Autodesk Inventor part; units mm, degrees
ref_plane "YZ Plane" through (0, 0, 0) normal (1, 0, 0) x (0, 1, 0)
ref_plane "XZ Plane" through (0, 0, 0) normal (0, 1, 0) x (-1, 0, 0)
ref_plane "XY Plane" through (0, 0, 0) normal (0, 0, 1) x (1, 0, 0)
sketch "Skizze1" plane through (0, 0, 0) normal (0, 0, 1) x (1, 0, 0)
  line L0 (-68.016, 1.808) -> (67.584, 1.808)
  line L1 (67.584, 1.808) -> (67.584, -2.192)
  line L2 (67.584, -2.192) -> (-68.016, -2.192)
  line L3 (-68.016, -2.192) -> (-68.016, 1.808)
  line L4 (-68.016, 1.808) -> (67.584, -2.192) construction
  line L5 (67.584, 1.808) -> (-68.016, -2.192) construction
  point P0 (0, 0)
  point P1 (-0.216, -0.192)
  point P2 (-0.216, -0.192)
  dimension "d0" = 135.6
  dimension "d1" = 4
extrude "Extrusion1" add sketch "Skizze1" along normal mid plane 3.25
ref_plane "Arbeitsebene1" through (-68.016, -0.192, 1.625) normal (0, -1, 0) x (1, 0, 0)
sketch "Skizze2" plane through (-68.016, -0.192, 1.625) normal (0, -1, 0) x (1, 0, 0)
  line L0 (0, -3.25) -> (0, 0)
  line L1 (0, -3.25) -> (135.6, -3.25)
  line L2 (0, 0) -> (2.85, 0)
  line L3 (2.85, 0) -> (2.85, -3.25)
  line L4 (2.85, -3.25) -> (0, -3.25)
  line L5 (0, -3.25) -> (0, 0)
  line L6 (0, 0) -> (0, 1.75)
  line L7 (0, 1.75) -> (2.85, 0)
  line L8 (135.6, -3.25) -> (135.6, 0)
  line L9 (135.6, 0) -> (132.75, 0)
  line L10 (132.75, 0) -> (132.75, -3.25)
  line L11 (132.75, -3.25) -> (135.6, -3.25)
  line L12 (135.6, -3.25) -> (135.6, 0)
  line L13 (135.6, 0) -> (135.6, 1.75)
  line L14 (135.6, 1.75) -> (132.75, 0)
  point P0 (68.016, -1.625)
  dimension "d4" = 2.85
  dimension "d5" = 1.75
  dimension "d6" = 2.85
extrude "Extrusion2" add sketch "Skizze2" along normal mid plane 19.7
sketch "Skizze3" plane through (0, 0, 1.625) normal (0, 0, 1) x (1, 0, 0)
  circle A0 centre (0, 0) radius 16
  dimension "d9" = 32
extrude "Extrusion3" cut sketch "Skizze3" against normal through all
sketch "Skizze4" plane through (0, 0, -1.625) normal (0, 0, -1) x (-1, 0, 0)
  line L0 (0.0777, -0.1628) -> (6.2277, -0.1628) construction
  circle A0 centre (0.0009, -0.1935) radius 13.625
  circle A1 centre (0.0009, -0.1935) radius 16.625
  line L1 (-22.383, -8.7935) -> (26.817, -8.7935)
  point P0 (-16.6241, -0.1935)
  point P1 (16.6259, -0.1935)
  point P2 (10.5688, -8.7935)
  point P3 (14.2287, -8.7935)
  point P4 (-14.2269, -8.7935)
  point P5 (-10.567, -8.7935)
  dimension "d27" = 3
  dimension "d28" = 27.25
  dimension "d29" = 8.6
extrude "Extrusion4" add sketch "Skizze4" against normal blind 6.5 contours A0 L1 A1 picked at (15.3303, 2.2297)
sketch "Skizze7" plane through (0, 0, 1.625) normal (0, 0, 1) x (1, 0, 0)
  line L0 (-65.166, 1.808) -> (-16.5049, 1.808)
  line L1 (-16.5053, -2.192) -> (-65.166, -2.192)
  line L2 (-16.5049, 1.808) -> (-61.5049, 1.808)
  line L3 (-61.5049, 1.808) -> (-61.5049, -2.192)
  line L4 (-61.5049, -2.192) -> (-16.5049, -2.192)
  line L5 (-16.5049, -2.192) -> (-16.5049, 1.808)
  line L6 (16.5032, 1.808) -> (64.734, 1.808)
  line L7 (64.734, -2.192) -> (16.5036, -2.192)
  line L8 (16.5032, 1.808) -> (61.5032, 1.808)
  line L9 (61.5032, 1.808) -> (61.5032, -2.192)
  line L10 (61.5032, -2.192) -> (16.5032, -2.192)
  line L11 (16.5032, -2.192) -> (16.5032, 1.808)
  point P0 (0, 0)
  point P1 (-61.5049, 1.808)
  point P2 (16.5036, -2.192)
  point P3 (61.5032, 1.808)
  dimension "d30" = 45
  dimension "d31" = 45
extrude "Extrusion7" add sketch "Skizze7" along normal blind 3.25
sketch "Skizze8" plane through (-65.166, -2.192, -1.625) normal (0, -1, 0) x (1, 0, 0)
  line L0 (48.661, 6.5) -> (3.661, 6.5)
  line L1 (48.661, 6.5) -> (48.661, 0)
  line L2 (3.661, 6.5) -> (48.661, 6.5)
  line L3 (48.661, 6.5) -> (48.661, 3.25)
  line L4 (48.661, 3.25) -> (3.661, 3.25)
  line L5 (3.661, 3.25) -> (3.661, 6.5)
  line L6 (126.6692, 3.25) -> (126.6692, 6.5)
  line L7 (81.6692, 6.5) -> (81.6692, 0)
  line L8 (126.6692, 6.5) -> (81.6692, 6.5)
  line L9 (81.6692, 6.5) -> (81.6692, 3.25)
  line L10 (81.6692, 3.25) -> (126.6692, 3.25)
  line L11 (126.6692, 3.25) -> (126.6692, 6.5)
  line L12 (81.6692, 6.5) -> (126.6692, 3.25)
  line L13 (50.9373, 6.5) -> (48.6607, 6.5)
  line L14 (48.6607, 6.5) -> (3.661, 3.25)
  point P0 (65.166, 1.625)
extrude "Extrusion8" cut sketch "Skizze8" against normal through all contours L14 L5 L0 | L12 L8 L6
properties part number "2024_08_28_Holder_GL25"
Read the model definition and answer for the solid it produces. Units are mm, in the model's axes. A direction names the side the tool comes from. Give positions to 0.01 mm unless a question says otherwise; leave off trailing zeros. Order: outer loops, then holes, each group sorted by start corner. A loop starts at its lowest first (then second) coordinate and runs counter-clockwise, first axis right, second up. Notation, with made-up numbers: (-31, 36.5) -> (5, 36.5) arc R28 cw to (5, 62.5) -> close; hole circle Ø4 at (-6.5, 88.5). An arc over 180 degrees is marked (long way). One line per item, written item: value. Start each with the question number.
(1) For a pull along X with two mould halves and no side action, classify faces 1 (the flat face through (-65.166, 6, 0)), 2 (the flat face through (12, -8.794, 2)), 3 (the flat face through (67.584, 0, 1)), 4 (the flat face through (66, 9.658, 0)) as released by +X, released by -X, zero draft, split by the parting line, or undercut.
(2) The part is cut by section C-C (y = -6.5). Determine the outline of the cut face in (x, z) (3 decimals), and give its area (3 significant figures).
(3) The part is cut by section D-D (x = 4). Determine the outline of the cut face in (y, z) (3 decimals).
(4) The part is cut by section B-B (y = -0.5). Determine the outline of the cut face in (x, z) (3 decimals).
(5) A tool of negligible diameter and unlimited length cuts with its end or side. For faces 5 (the flat face through (10.14, 9.14, -1.625)), 6 (the flat face through (38.688, -0.22, 3.273)), 7 (the flat face through (-40, -2.192, 1)), 8 (the flat face through (-41, 1.808, 1)), from which of +Z, -Z, +X, -X, +Y, -Y can it reach the whole face along a straight path? Write none if from no direction.
(6) Flat-ended cylindrical pins translate along their axes: P1, Ø3.5, axis at x = 30.5, z = 0, coming from the +Y side; P2, Ø1.6, axis at x = 62.5, y = 0.5, coming from the +Z side (3 decimals); P3, Ø3, axis at x = -66, z = 0, coming from the +Y side. Find the tip coordinate at first contact, or state that the pin passes through.
(7) Straight lines are drawn through the part: L1, parallel to X at y = 0, z = 1; L2, parallel to X at y = 4, z = 0; L3, parallel to X at y = 3, z = 3. For each, find the intervals that lie inside material, in ascending order.
Taken from the geometry:
1. face 1: undercut
1. face 2: undercut
1. face 3: released by +X
1. face 4: zero draft
2. outline: (-68.016, -1.625) -> (-65.166, -1.625) -> (-65.166, 1.625) -> (-68.016, 3.375) -> close; (-15.383, -1.625) -> (-12.079, -1.625) -> (-12.079, 4.875) -> (-15.383, 4.875) -> close; (12.077, -1.625) -> (15.382, -1.625) -> (15.382, 4.875) -> (12.077, 4.875) -> close; (64.734, -1.625) -> (67.584, -1.625) -> (67.584, 3.375) -> (64.734, 1.625) -> close
2. area: 66.5 mm^2
3. outline: (12.831, -1.625) -> (15.943, -1.625) -> (15.943, 4.875) -> (12.831, 4.875) -> close
4. outline: (-68.016, -1.625) -> (-13.622, -1.625) -> (-13.622, 4.875) -> (-16.505, 4.875) -> (-61.505, 1.625) -> (-65.166, 1.625) -> (-68.016, 3.375) -> close; (13.621, -1.625) -> (67.584, -1.625) -> (67.584, 3.375) -> (64.734, 1.625) -> (61.503, 1.625) -> (16.503, 4.875) -> (13.621, 4.875) -> close
5. face 5: -Z, +X, -X, +Y, -Y
5. face 6: +Z, +Y, -Y
5. face 7: +Z, -Z, -Y
5. face 8: +Z, -Z, +Y
6. P1: y = 1.81
6. P2: z = 1.625
6. P3: y = 9.66
7. L1: -68.02 to -13.62, 13.62 to 67.58
7. L2: -68.02 to -65.17, -16.09 to -12.96, 12.96 to 16.09, 64.73 to 67.58
7. L3: -68.02 to -67.41, -16.32 to -13.25, 13.24 to 16.31, 66.97 to 67.58
